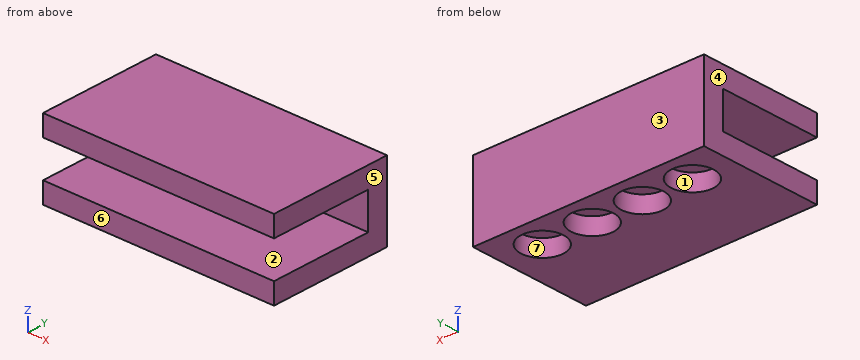
```python
from build123d import *

# Parameters (mm, degrees)
SKETCH2_W           = 36
SKETCH2_H           = 19.2
BOSS_EXTRUDE1_DEPTH = 5.994
SKETCH3_W           = 36
SKETCH3_H           = 16
CUT_EXTRUDE1_DEPTH  = 2.794
SKETCH4_R           = 3.3
CUT_EXTRUDE2_DEPTH  = 2.6


with BuildPart() as part:
    # Sketch2 → Boss-Extrude1 (new, symmetric)
    with BuildSketch(Plane.XY):
        with Locations((0, -6.4)):
            Rectangle(SKETCH2_W, SKETCH2_H)
    extrude(amount=BOSS_EXTRUDE1_DEPTH, both=True)

    # Sketch3 → Cut-Extrude1 (cut, symmetric)
    with BuildSketch(Plane.XY):
        with Locations((0, -8)):
            Rectangle(SKETCH3_W, SKETCH3_H)
    extrude(amount=CUT_EXTRUDE1_DEPTH, both=True, mode=Mode.SUBTRACT)

    # Sketch4 → Cut-Extrude2 (cut)
    with BuildSketch(Plane.XY.offset(-5.994)):
        with Locations((11.7, -1.7)):
            Circle(SKETCH4_R)
        with Locations((3.9, -1.7)):
            Circle(SKETCH4_R)
        with Locations((-3.9, -1.7)):
            Circle(SKETCH4_R)
        with Locations((-11.7, -1.7)):
            Circle(SKETCH4_R)
    extrude(amount=CUT_EXTRUDE2_DEPTH, mode=Mode.SUBTRACT)


solid = part.part
```
The listing builds one solid part. Answer for the finished solid, in the listing's coordinates (mm). Face numbers are marked on the shaded views. A direction names the side the tool comes from. Give positions to 0.01 mm unless a question says otherwise; leave off trailing zeros. Loops run counter-clockwise (first coordinate to the right, second up) from the corner with the lowest first, then second, coordinate; pieces in that order, holes last. Notation, with made-up numbers: (23.5, 70.5) - (52.5, 70.5) arc R16 cw to (52.5, 82.5) - close; hole circle Ø9 at (72.5, -16). An arc over 180 degrees is marked (long way). Answer as CSV lines item,"result". Start each with the question number.
Item 1: A cutting plane is placed at D-D on y = -6. Determine the outline of the cut face in (x, z), then the cut area to 3 significant figures.
Item 2: A cutting plane is placed at C-C on z = -0.75. Determine the outline of the cut face in (x, y), then the cut area to 3 significant figures.
Item 3: A cutting plane is placed at A-A on y = -1.7. Determine the outline of the cut face in (x, z), then the cut area to 3 significant figures.
Item 4: For the marked faces 1, 2 and 3, determine the directions among +Z, -Z, +X, -X, +Y, -Y from which every point of the face is accessible in a straight line to the end or side of a thin tool.
Item 5: Each of these flat-tipped pins is pushed along its axis until it touches: pin 1 (3.5 mm diameter, centred on x = 3.5, y = -2, fed in from -Z); pin 2 (3 mm diameter, centred on x = -3.5, z = 0.5, fed in from -Y). Where does it stop, or does it pass through?
Item 6: A cutting plane is placed at B-B on x = 11.7. Determine the outline of the cut face in (y, z).
Item 7: The mould has two halves that part along X. Classify the marked faces 4, 5, 6 and 7: +X half, -X half, draft (parallel to the pull), parting line (faces both ways), or undercut.
Item 8: Find the intervals of material crossed by line 1 (Z direction, x = 11.5, y = -3); line 2 (Z direction, x = -8.5, y = -8); line 3 (Y direction, x = 11.7, z = -4.85), in increasing order. Write a range as from..to.
Found:
1,outline,"(-18, -5.99) - (18, -5.99) - (18, -2.79) - (-18, -2.79) - close; (-18, 2.79) - (18, 2.79) - (18, 5.99) - (-18, 5.99) - close"
1,area,"230 mm^2"
2,outline,"(-18, 0) - (18, 0) - (18, 3.2) - (-18, 3.2) - close"
2,area,"115 mm^2"
3,outline,"(-18, -5.99) - (-15, -5.99) - (-15, -3.39) - (-8.4, -3.39) - (-8.4, -5.99) - (-7.2, -5.99) - (-7.2, -3.39) - (-0.6, -3.39) - (-0.6, -5.99) - (0.6, -5.99) - (0.6, -3.39) - (7.2, -3.39) - (7.2, -5.99) - (8.4, -5.99) - (8.4, -3.39) - (15, -3.39) - (15, -5.99) - (18, -5.99) - (18, -2.79) - (-18, -2.79) - close; (-18, 2.79) - (18, 2.79) - (18, 5.99) - (-18, 5.99) - close"
3,area,"162 mm^2"
4,face 1,"-Z"
4,face 2,"+X, -X, -Y"
4,face 3,"+Z, -Z, +X, -X, +Y"
5,pin 1,"stops at z = -3.39"
5,pin 2,"stops at y = 0"
6,outline,"(-16, -5.99) - (-5, -5.99) - (-5, -3.39) - (1.6, -3.39) - (1.6, -5.99) - (3.2, -5.99) - (3.2, 5.99) - (-16, 5.99) - (-16, 2.79) - (0, 2.79) - (0, -2.79) - (-16, -2.79) - close"
7,face 4,"-X half"
7,face 5,"+X half"
7,face 6,"draft"
7,face 7,"undercut"
8,line 1,"z = -3.39..-2.79, 2.79..5.99"
8,line 2,"z = -5.99..-2.79, 2.79..5.99"
8,line 3,"y = -16..-5, 1.6..3.2"
